Design review of the part built by this model. Coordinates are the model's own, in mm. Give positions to 0.01 mm unless a question says otherwise; leave off trailing zeros. Order: outer loops, then holes, each group sorted by start corner. A loop starts at its lowest first (then second) coordinate and runs counter-clockwise, first axis right, second up. Notation, with made-up numbers: (69.25, -32.75) -> (101.25, -32.75) arc R24 ccw to (101.25, -1.75) -> close; hole circle Ø3 at (50.5, -17.5). An arc over 180 degrees is marked (long way). Answer in a Markdown table with one row per item. Add a question column.
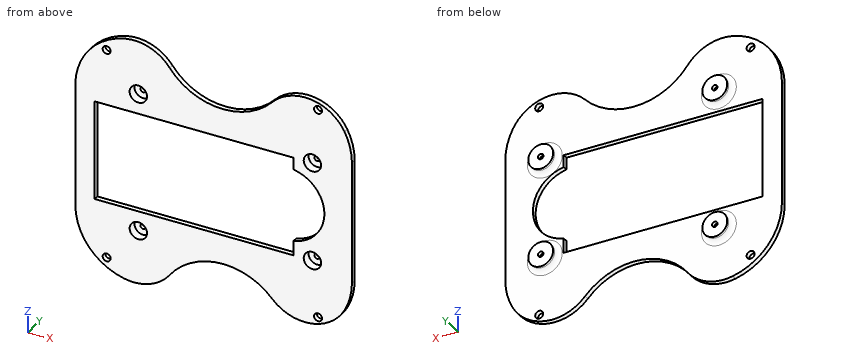
```python
from build123d import *

# Parameters (mm, degrees)
SKETCH1_W               = 111.193579624
SKETCH1_H               = 99.509273796
SKETCH1_R               = 1.6
BOSS_EXTRUDE1_DEPTH     = 2
SKETCH2_R               = 5
BOSS_EXTRUDE2_DEPTH     = 3
CUT_EXTRUDE2_DEPTH      = 75.776513226
CUT_EXTRUDE2_DEPTH_BACK = 75.776513226
SKETCH3_R               = 1.1
CUT_EXTRUDE3_DEPTH      = 75.776513226
CUT_EXTRUDE3_DEPTH_BACK = 3.5
SKETCH4_R               = 3.5
FILLET1_R               = 25
CUT_EXTRUDE4_DEPTH      = 75.669451118
CUT_EXTRUDE4_DEPTH_BACK = 75.669451118
SKETCH5_W               = 80
SKETCH5_H               = 40
CUT_EXTRUDE5_DEPTH      = 75.669451118
CUT_EXTRUDE5_DEPTH_BACK = 75.669451118
CUT_EXTRUDE6_DEPTH      = 75.669451118
CUT_EXTRUDE6_DEPTH_BACK = 75.669451118
FILLET3_R               = 2
FILLET4_R               = 18


with BuildPart() as part:
    # Sketch1 → Boss-Extrude1 (new body)
    with BuildSketch(Plane(origin=(0, 0, 0), x_dir=(1, 0, 0), z_dir=(0, 1, 0))):
        Rectangle(SKETCH1_W, SKETCH1_H)
        with Locations(Location((-43.005863497, 42.538435101, 0), (0, 0, 270))):
            Circle(SKETCH1_R, mode=Mode.SUBTRACT)
        with Locations(Location((41.994136503, 42.538435101, 0), (0, 0, 270))):
            Circle(SKETCH1_R, mode=Mode.SUBTRACT)
        with Locations(Location((41.994136503, -42.461564899, 0), (0, 0, 270))):
            Circle(SKETCH1_R, mode=Mode.SUBTRACT)
        with Locations(Location((-43.005863497, -42.461564899, 0), (0, 0, 270))):
            Circle(SKETCH1_R, mode=Mode.SUBTRACT)
    extrude(amount=BOSS_EXTRUDE1_DEPTH)

    # Sketch2 → Boss-Extrude2 (add)
    with BuildSketch(Plane(origin=(0, 2, 0), x_dir=(1, 0, 0), z_dir=(0, 1, 0))):
        with Locations(Location((-30.275730538, 27.936106549, 0), (0, 0, 270))):
            Circle(SKETCH2_R)
        with Locations(Location((39.724269462, 19.936106549, 0), (0, 0, 270))):
            Circle(SKETCH2_R)
        with Locations(Location((39.724269462, -20.063893451, 0), (0, 0, 270))):
            Circle(SKETCH2_R)
        with Locations(Location((-30.275730538, -28.063893451, 0), (0, 0, 270))):
            Circle(SKETCH2_R)
    extrude(amount=BOSS_EXTRUDE2_DEPTH)

    # Sketch3 → Cut-Extrude2 (cut, two sides: drawn at the far end of the back side and taken through both)
    with BuildSketch(Plane(origin=(0, 5, 0), x_dir=(1, 0, 0), z_dir=(0, 1, 0)).offset(-CUT_EXTRUDE2_DEPTH_BACK)):
        with Locations(Location((-30.275730538, 27.936106549, 0), (0, 0, 270))):
            Circle(SKETCH3_R)
        with Locations(Location((39.724269462, 19.936106549, 0), (0, 0, 270))):
            Circle(SKETCH3_R)
        with Locations(Location((39.724269462, -20.063893451, 0), (0, 0, 270))):
            Circle(SKETCH3_R)
        with Locations(Location((-30.275730538, -28.063893451, 0), (0, 0, 270))):
            Circle(SKETCH3_R)
    extrude(amount=CUT_EXTRUDE2_DEPTH + CUT_EXTRUDE2_DEPTH_BACK, mode=Mode.SUBTRACT)

    # Sketch4 → Cut-Extrude3 (cut, two sides: drawn at the far end of the back side and taken through both)
    with BuildSketch(Plane.XZ.offset(-CUT_EXTRUDE3_DEPTH_BACK)):
        with Locations(Location((-30.275730538, 28.063893451, 0), (0, 0, 90))):
            Circle(SKETCH4_R)
        with Locations(Location((39.724269462, 20.063893451, 0), (0, 0, 90))):
            Circle(SKETCH4_R)
        with Locations(Location((39.724269462, -19.936106549, 0), (0, 0, 90))):
            Circle(SKETCH4_R)
        with Locations(Location((-30.275730538, -27.936106549, 0), (0, 0, 90))):
            Circle(SKETCH4_R)
    extrude(amount=CUT_EXTRUDE3_DEPTH + CUT_EXTRUDE3_DEPTH_BACK, mode=Mode.SUBTRACT)

    # Fillet1
    fillet1_edges = [part.edges().sort_by_distance(p)[0] for p in [
        (-55.596789812, 1, -49.754636898),
        (55.596789812, 1, -49.754636898),
        (55.596789812, 1, 49.754636898),
        (-55.596789812, 1, 49.754636898),
    ]]
    fillet(fillet1_edges, radius=FILLET1_R)

    # Sketch5 → Cut-Extrude4 (cut, two sides: drawn at the far end of the back side and taken through both)
    with BuildSketch(Plane(origin=(0, 2, 0), x_dir=(1, 0, 0), z_dir=(0, 1, 0)).offset(-CUT_EXTRUDE4_DEPTH_BACK)):
        with Locations((-7.838338825, 0)):
            Rectangle(SKETCH5_W, SKETCH5_H)
    extrude(amount=CUT_EXTRUDE4_DEPTH + CUT_EXTRUDE4_DEPTH_BACK, mode=Mode.SUBTRACT)

    # Sketch6 → Cut-Extrude5 (cut, two sides: drawn at the far end of the back side and taken through both)
    with BuildSketch(Plane(origin=(0, 2, 0), x_dir=(1, 0, 0), z_dir=(0, 1, 0)).offset(-CUT_EXTRUDE5_DEPTH_BACK)):
        with BuildLine():
            Line((-21.585028243, -49.754636898), (29.257650702, -49.754636898))
            ThreePointArc((29.257650702, -49.754636898), (3.836311229, -31.705915293), (-21.585028243, -49.754636898))
        make_face()
        with BuildLine():
            Line((-21.585028243, 49.754636898), (29.257650702, 49.754636898))
            ThreePointArc((29.257650702, 49.754636898), (3.836311229, 31.705915293), (-21.585028243, 49.754636898))
        make_face()
    extrude(amount=CUT_EXTRUDE5_DEPTH + CUT_EXTRUDE5_DEPTH_BACK, mode=Mode.SUBTRACT)

    # Sketch7 → Cut-Extrude6 (cut, two sides: drawn at the far end of the back side and taken through both)
    with BuildSketch(Plane(origin=(0, 2, 0), x_dir=(1, 0, 0), z_dir=(0, 1, 0)).offset(-CUT_EXTRUDE6_DEPTH_BACK)):
        with BuildLine():
            Line((32.161661175, 14.041836801), (32.161661175, -15.135059457))
            ThreePointArc((32.161661175, -15.135059457), (44.520164004, -0.546611328), (32.161661175, 14.041836801))
        make_face()
    extrude(amount=CUT_EXTRUDE6_DEPTH + CUT_EXTRUDE6_DEPTH_BACK, mode=Mode.SUBTRACT)

    # Fillet3
    fillet3_edges = [part.edges().sort_by_distance(p)[0] for p in [
        (-30.275730538, 2, -32.936106549),
        (39.724269462, 2, -24.936106549),
        (39.724269462, 2, 15.063893451),
        (-30.275730538, 2, 23.063893451),
    ]]
    fillet(fillet3_edges, radius=FILLET3_R)

    # Fillet4
    fillet4_edges = [part.edges().sort_by_distance(p)[0] for p in [
        (-21.585028243, 1, 49.754636898),
        (29.257650702, 1, 49.754636898),
        (29.257650702, 1, -49.754636898),
        (-21.585028243, 1, -49.754636898),
    ]]
    fillet(fillet4_edges, radius=FILLET4_R)


solid = part.part
```
1) Add section B-B, the plane z = -0.5. Write out the cut boundary in (x, y).
2) Clearance check with flat-ended pins moving along their axes: P1, Ø1.6, axis at x = 8.5, y = 1, coming from the +Z side; P2, Ø3.5, axis at x = -43.01, z = 42.46, coming from the +Y side; P3, Ø2, axis at y = 4, z = 39, coming from the +X side; P4, Ø2, axis at x = 6, y = 1.5, coming from the +Z side. State where each tip first meets the part, or that it passes through.
3) Add section A-A, the plane x = 12. Write out the cut boundary in (y, z).
4) Add section C-C, the plane y = 1. Give the number of separate pieces and of enclosed holes in the cut face, and give its area (3 significant figures).
5) For L1, parallel to Z at x = 39.5, y = 0.6; L2, parallel to Z at x = -33, y = 1.2; L3, parallel to Y at x = 31, z = -34.5, list the stretches that pass through material, from the lowest coordinate up.
Verdict:
| question | item | result |
|---|---|---|
| 1 | outline | (-55.6, 0) -> (-47.84, 0) -> (-47.84, 2) -> (-55.6, 2) -> close; (44.48, 0) -> (55.6, 0) -> (55.6, 2) -> (44.48, 2) -> close |
| 2 | P1 | stops at z = 32.27 |
| 2 | P2 | stops at y = 2 |
| 2 | P3 | passes through |
| 2 | P4 | stops at z = 31.89 |
| 3 | outline | (0, -32.97) -> (2, -32.97) -> (2, -20) -> (0, -20) -> close; (0, 20) -> (2, 20) -> (2, 32.97) -> (0, 32.97) -> close |
| 4 | separate pieces | 1 |
| 4 | enclosed holes | 9 |
| 4 | area | 5,380 mm2 |
| 5 | L1 | z = -45.86 to -23.43, -16.44 to -10.56, 11.65 to 16.57, 23.56 to 45.86 |
| 5 | L2 | z = -49.58 to -30.13, -25.74 to -20, 20 to 25.87, 30.26 to 49.58 |
| 5 | L3 | y = 0 to 2 |
